The listing builds one solid part. Answer for the finished solid, in the listing's coordinates (mm). Face numbers are marked on the shaded views. A direction names the side the tool comes from. Give positions to 0.01 mm unless a question says otherwise; leave off trailing zeros. Write each loop counter-clockwise with the first axis right and the second up, starting at its lowest first coordinate (ties: lowest second). Pieces come first, ordered by that corner, then holes. Notation, with made-up numbers: (-30.5, 17.5) - (-23.5, 17.5) arc R33 cw to (-23.5, 48.5) - close; hole circle Ø11 at (5, -5). An arc over 180 degrees is marked (long way). Answer in a Markdown table with one row per item. Add a question column.
from build123d import *

# Parameters (mm, degrees)
SKETCH_1_W          = 120
SKETCH_1_H          = 50
EXTRUDE_1_DEPTH     = 14
EXTRUDE_START       = -20
EXTRUDE_3_DEPTH     = 40
SKETCH_4_R          = 17.5
CUT_EXTRUDE_1_DEPTH = 112.803398875
SKETCH_5_W          = 60
SKETCH_5_H          = 50
CUT_EXTRUDE_2_DEPTH = 3
SKETCH_6_R          = 6
CUT_EXTRUDE_3_DEPTH = 93.633687177
SKETCH_7_R          = 3
CUT_EXTRUDE_4_DEPTH = 13


# Read off the part's stored shape, not the designer's step: 凸台-拉伸3
with BuildPart() as part:
    # 草图1 → 凸台-拉伸1 (new body)
    with BuildSketch(Plane(origin=(0, 0, 0), x_dir=(1, 0, 0), z_dir=(0, 1, 0))):
        Rectangle(SKETCH_1_W, SKETCH_1_H)
    extrude(amount=EXTRUDE_1_DEPTH)

    # 凸台-拉伸3 outline → 凸台-拉伸3 (add)
    with BuildSketch(Plane.XY.offset(EXTRUDE_START)):
        with BuildLine():
            Line((30, 14), (30, 50))
            ThreePointArc((30, 50), (0, 80), (-30, 50))
            Line((-30, 50), (-30, 14))
            Line((-30, 14), (30, 14))
        make_face()
    extrude(amount=EXTRUDE_3_DEPTH)

    # 草图4 → 切除-拉伸1 (cut, through all)
    with BuildSketch(Plane.XY.offset(25)):
        with Locations(Location((0, 50, 0), (0, 0, 180))):
            Circle(SKETCH_4_R)
    extrude(amount=-CUT_EXTRUDE_1_DEPTH, mode=Mode.SUBTRACT)

    # 草图5 → 切除-拉伸2 (cut)
    with BuildSketch(Plane(origin=(0, 0, 0), x_dir=(1, 0, 0), z_dir=(0, 1, 0))):
        Rectangle(SKETCH_5_W, SKETCH_5_H)
    extrude(amount=CUT_EXTRUDE_2_DEPTH, mode=Mode.SUBTRACT)

    # 草图6 → 切除-拉伸3 (cut, through all)
    with BuildSketch(Plane(origin=(0, 14, 0), x_dir=(1, 0, 0), z_dir=(0, 1, 0))):
        with Locations(Location((-45, 0, 0), (0, 0, 270))):
            Circle(SKETCH_6_R)
        with Locations(Location((45, 0, 0), (0, 0, 270))):
            Circle(SKETCH_6_R)
    extrude(amount=-CUT_EXTRUDE_3_DEPTH, mode=Mode.SUBTRACT)

    # 草图7 → 切除-拉伸4 (cut)
    with BuildSketch(Plane(origin=(0, 80, 0), x_dir=(1, 0, 0), z_dir=(0, 1, 0))):
        with Locations(Location((0, 0, 0), (0, 0, 270))):
            Circle(SKETCH_7_R)
    extrude(amount=-CUT_EXTRUDE_4_DEPTH, mode=Mode.SUBTRACT)


solid = part.part
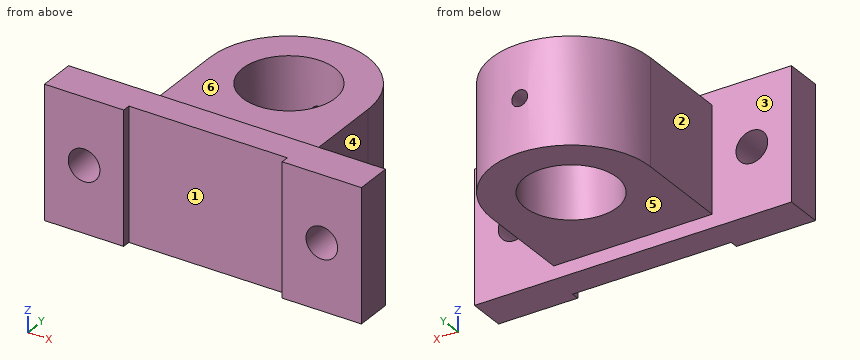
1. Section C-C (y = 66) is taken. Give the vertices of the cut face in (x, z), and give its area (3 significant figures).
2. Section B-B (z = 18.5) is taken. Give the vertices of the cut face in (x, y).
3. Given pin 1 Ø18 at (x, y) = (-5.5, 60) entering from -Z; pin 2 Ø1.5 at (y, z) = (27.5, -11.5) entering from -X; pin 3 Ø5 at (y, z) = (49.5, 10) entering from +X, each flat-ended and moving along its own axis, determine where each tip first touches the part or whether it passes through.
4. Section D-D (z = 0) is taken. Give the vertices of the cut face in (x, y).
5. The mould has two halves that part along X. Classify the marked faces 1, 2 and 3: +X half, -X half, draft (parallel to the pull), parting line (faces both ways), or undercut.
6. Section A-A (x = 0) is taken. Give the vertices of the cut face in (y, z), and give its area (4 significant figures).
7. A tool of negligible diameter and unlimited length cuts with its end or side. For the marked faces 4, 5 and 6, from which of +Z, -Z, +X, -X, +Y, -Y can it reach the whole face along a straight path? Write none if from no direction.
8. Straight lines are drawn through the part: L1, parallel to X at y = 7, z = 0; L2, parallel to Z at x = 0, y = 71.5; L3, parallel to X at y = 50, z = -8. For each, find the intervals that lie inside material, in ascending order. Write a range as [from, to].
Geometry check:
| question | item | result |
|---|---|---|
| 1 | outline | (-25.38, -20) - (-7.09, -20) - (-7.09, 20) - (-25.38, 20) - close; (7.09, -20) - (25.38, -20) - (25.38, 20) - (7.09, 20) - close |
| 1 | area | 1,460 mm² |
| 2 | outline | (-60, 0) - (-30, 0) - (-30, 3) - (30, 3) - (30, 0) - (60, 0) - (60, 14) - (30, 14) - (30, 50) arc R30 ccw to (-30, 50) - (-30, 14) - (-60, 14) - close; hole circle Ø35 at (0, 50) |
| 3 | pin 1 | z = -20 |
| 3 | pin 2 | x = -30 |
| 3 | pin 3 | x = 30 |
| 4 | outline | (-60, 0) - (-51, 0) - (-51, 14) - (-60, 14) - close; (-39, 0) - (-30, 0) - (-30, 3) - (30, 3) - (30, 0) - (39, 0) - (39, 14) - (30, 14) - (30, 50) arc R30 ccw to (3, 79.85) - (3, 67.24) arc R17.5 cw (long way) to (-3, 67.24) - (-3, 79.85) arc R30 ccw to (-30, 50) - (-30, 14) - (-39, 14) - close; (51, 0) - (60, 0) - (60, 14) - (51, 14) - close |
| 5 | face 1 | undercut |
| 5 | face 2 | -X half |
| 5 | face 3 | draft |
| 6 | outline | (3, -25) - (14, -25) - (14, -20) - (32.5, -20) - (32.5, 20) - (14, 20) - (14, 25) - (3, 25) - close; (67.5, -20) - (80, -20) - (80, -3) - (67.5, -3) - close; (67.5, 3) - (80, 3) - (80, 20) - (67.5, 20) - close |
| 6 | area | 1,715 mm² |
| 7 | face 4 | +Z, -Z, +X, +Y |
| 7 | face 5 | -Z, +X, -X, +Y |
| 7 | face 6 | +Z, +X, -X, +Y |
| 8 | L1 | [-60, -51], [-39, 39], [51, 60] |
| 8 | L2 | [-20, -3], [3, 20] |
| 8 | L3 | [-30, -17.5], [17.5, 30] |
